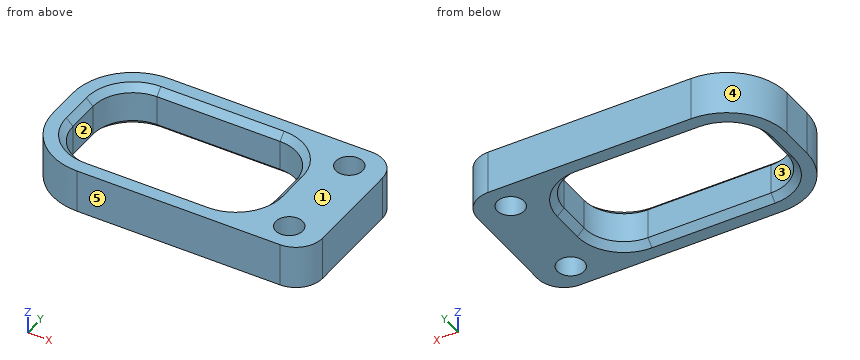
from build123d import *

# Parameters (mm, degrees)
SKETCH1_R           = 2.025483479
BOSS_EXTRUDE1_DEPTH = 6.5
CHAMFER1_SIZE       = 1


with BuildPart() as part:
    # Sketch1 → Boss-Extrude1 (new body)
    with BuildSketch(Plane.XY):
        with BuildLine():
            Line((-29.5, 4), (1, 4))
            ThreePointArc((1, 4), (3.828427125, 2.828427125), (5, 0))
            Line((5, 0), (5, -15))
            ThreePointArc((5, -15), (3.828427125, -17.828427125), (1, -19))
            Line((1, -19), (-29.5, -19))
            ThreePointArc((-29.5, -19), (-35.863961031, -16.363961031), (-38.5, -10))
            Line((-38.5, -10), (-38.5, -5))
            ThreePointArc((-38.5, -5), (-35.863961031, 1.363961031), (-29.5, 4))
        make_face()
        Circle(SKETCH1_R, mode=Mode.SUBTRACT)
        with Locations((0, -15)):
            Circle(SKETCH1_R, mode=Mode.SUBTRACT)
        with BuildLine():
            Line((-29.5, 1), (-11, 1))
            ThreePointArc((-11, 1), (-6.757359313, -0.757359313), (-5, -5))
            Line((-5, -5), (-5, -10))
            ThreePointArc((-5, -10), (-6.757359313, -14.242640687), (-11, -16))
            Line((-11, -16), (-29.5, -16))
            ThreePointArc((-29.5, -16), (-33.742640687, -14.242640687), (-35.5, -10))
            Line((-35.5, -10), (-35.5, -5))
            ThreePointArc((-35.5, -5), (-33.742640687, -0.757359313), (-29.5, 1))
        make_face(mode=Mode.SUBTRACT)
    extrude(amount=BOSS_EXTRUDE1_DEPTH)

    # Chamfer1
    chamfer1_edges = [part.edges().sort_by_distance(p)[0] for p in [
        (-6.757359313, -0.757359313, 0),
        (-20.25, 1, 0),
        (-33.742640687, -0.757359313, 0),
        (-35.5, -7.5, 0),
        (-33.742640687, -14.242640687, 0),
        (-20.25, -16, 0),
        (-6.757359313, -14.242640687, 0),
        (-5, -7.5, 0),
        (-6.757359313, -0.757359313, 6.5),
        (-20.25, 1, 6.5),
        (-33.742640687, -0.757359313, 6.5),
        (-35.5, -7.5, 6.5),
        (-33.742640687, -14.242640687, 6.5),
        (-20.25, -16, 6.5),
        (-6.757359313, -14.242640687, 6.5),
        (-5, -7.5, 6.5),
    ]]
    chamfer(chamfer1_edges, length=CHAMFER1_SIZE)


solid = part.part
Source: CAD feature listing. Evaluate the final solid. Frame: model axes, mm. Face numbers are marked on the shaded views. A direction names the side the tool comes from. Round coordinates to 2 decimals unless told otherwise and drop trailing zeros. Loops run counter-clockwise (first coordinate to the right, second up) from the corner with the lowest first, then second, coordinate; pieces in that order, holes last. Notation, with made-up numbers: M 68,2.25 L 95,2.25 A16 ccw 95,31.25 Z; hole C 73,-37 d6. An arc over 180 degrees is marked long. Return JSON: item names as keys, results as strings. Group by question number.
1. Pin query (flat end, axial travel): pin 1 (3 mm diameter, centred on x = 0, y = 0, fed in from -Z); pin 2 (3 mm diameter, centred on x = -6, y = -3.5, fed in from -Z); pin 3 (1 mm diameter, centred on x = -32.5, z = 2.5, fed in from +Y); pin 4 (1 mm diameter, centred on y = -15, z = 1.5, fed in from -X). Return the tip coordinate at first contact, or that it passes through.
2. Section query B-B on x = -29. Output: boundary loops of the cut face in (y, z), and give its area (3 significant figures).
3. Section query C-C on x = 0. Output: boundary loops of the cut face in (y, z).
4. Section query A-A on z = 6. Output: boundary loops of the cut face in (x, y).
5. Section query D-D on z = 3. Output: boundary loops of the cut face in (x, y), and give its area (3 significant figures).
6. Reachability of the marked faces 1 and 2 from +Z, -Z, +X, -X, +Y, -Y: full face, straight path, thin tool, end or side. Return the list, or none.
7. Mould query, pull axis Y, two halves, no side actions, for the marked faces 3, 4 and 5. Classes: released by +Y, released by -Y, zero draft, split by the parting line, or undercut.
8. Material intervals for line 1 along Y through (x, z) = (0, 2.5); line 2 along Y through (x, z) = (-29, 1.5); line 3 along X through (y, z) = (-1.5, 5), sorted ascending. Write a range as from..to.
Checks:
{
 "1": {"pin 1": "passes through", "pin 2": "stops at z = 0.28", "pin 3": "stops at y = 3.65", "pin 4": "stops at x = -37.29"},
 "2": {"outline": "M -19,0 L -17,0 L -16,1 L -16,5.5 L -17,6.5 L -19,6.5 Z; M 1,1 L 2,0 L 4,0 L 4,6.5 L 2,6.5 L 1,5.5 Z", "area": "37.0 mm²"},
 "3": {"outline": "M -19,0 L -17.03,0 L -17.03,6.5 L -19,6.5 Z; M -12.97,0 L -2.03,0 L -2.03,6.5 L -12.97,6.5 Z; M 2.03,0 L 4,0 L 4,6.5 L 2.03,6.5 Z"},
 "4": {"outline": "M -38.5,-10 A9 ccw -29.5,-19 L 1,-19 A4 ccw 5,-15 L 5,0 A4 ccw 1,4 L -29.5,4 A9 ccw -38.5,-5 Z; hole M -36,-10 A6.5 ccw -29.5,-16.5 L -11,-16.5 A6.5 ccw -4.5,-10 L -4.5,-5 A6.5 ccw -11,1.5 L -29.5,1.5 A6.5 ccw -36,-5 Z; hole C 0,-15 d4.05; hole C 0,0 d4.05"},
 "5": {"outline": "M -38.5,-10 A9 ccw -29.5,-19 L 1,-19 A4 ccw 5,-15 L 5,0 A4 ccw 1,4 L -29.5,4 A9 ccw -38.5,-5 Z; hole M -35.5,-10 A6 ccw -29.5,-16 L -11,-16 A6 ccw -5,-10 L -5,-5 A6 ccw -11,1 L -29.5,1 A6 ccw -35.5,-5 Z; hole C 0,-15 d4.05; hole C 0,0 d4.05", "area": "445 mm²"},
 "6": {"face 1": "+Z, +X, -X, +Y, -Y", "face 2": "+Z, -Z"},
 "7": {"face 3": "undercut", "face 4": "released by +Y", "face 5": "released by -Y"},
 "8": {"line 1": "y = -19..-17.03, -12.97..-2.03, 2.03..4", "line 2": "y = -19..-16, 1..4", "line 3": "x = -37.79..-34.37, -6.13..-1.36, 1.36..5"}
}
